```python
from build123d import *

# Parameters (mm, degrees)
BOX018_W     = 173
BOX018_H     = 97.5
BOX018_DEPTH = 30
BOX019_W     = 181
BOX019_H     = 121
BOX019_DEPTH = 5
BOX017_W     = 186
BOX017_H     = 127
BOX017_DEPTH = 2
FILLET008_R  = 2
FILLET009_R  = 1


with BuildPart() as cutout:
    # Box018 → Box018 (new body)
    with BuildSketch(Plane(origin=(6.5, 11, -25), x_dir=(1, 0, 0), z_dir=(0, 0, 1))):
        with Locations((86.5, 48.75)):
            Rectangle(BOX018_W, BOX018_H)
    extrude(amount=BOX018_DEPTH)


with BuildPart() as cube016:
    # Box019 → Box019 (new body)
    with BuildSketch(Plane(origin=(2.5, 3, -5), x_dir=(1, 0, 0), z_dir=(0, 0, 1))):
        with Locations((90.5, 60.5)):
            Rectangle(BOX019_W, BOX019_H)
    extrude(amount=BOX019_DEPTH)


with BuildPart() as fascia:
    # Box017 → Box017 (new body)
    with BuildSketch(Plane.XY):
        with Locations((93, 63.5)):
            Rectangle(BOX017_W, BOX017_H)
    extrude(amount=BOX017_DEPTH)

    # Fusion007: union Cube016
    add(cube016.part)

    # Cut007: cut Cutout
    add(cutout.part, mode=Mode.SUBTRACT)

    # Fillet008
    fillet008_edges = [fascia.edges().sort_by_distance(p)[0] for p in [
        (2.5, 124, -2.5),
        (2.5, 63.5, -5),
        (93, 3, -5),
        (183.5, 63.5, -5),
    ]]
    fillet(fillet008_edges, radius=FILLET008_R)

    # Fillet009
    fillet009_edges = [fascia.edges().sort_by_distance(p)[0] for p in [
        (2.973408, 123.292098, -4.292098),
        (93, 3, -3),
        (183.5, 124, -1.5),
        (0, 0, 1),
        (0, 127, 1),
        (186, 127, 1),
        (186, 0, 1),
        (186, 63.5, 2),
    ]]
    fillet(fillet009_edges, radius=FILLET009_R)


solid = fascia.part
```
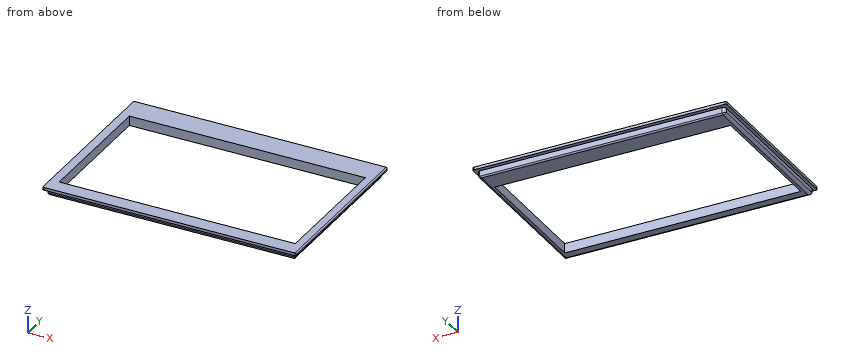
Source: CAD feature listing. Evaluate the final solid. Frame: model axes, mm. Coordinates: 2 decimals unless noted, no trailing zeros. Loops run counter-clockwise (first coordinate to the right, second up) from the corner with the lowest first, then second, coordinate; pieces in that order, holes last. Notation, with made-up numbers: (47.25, 56.25) -> (70.25, 56.25) arc R17 ccw to (70.25, 83.25) -> close; hole circle Ø2 at (70.5, 2.25). An arc over 180 degrees is marked (long way). One line per item, written item: value. Start each with the question number.
Q1. Contact query for flat-ended pins moving along their axis: P1, Ø1.2, axis at x = 86, z = -2.5, coming from the +Y side; P2, Ø1.5, axis at x = 42.5, z = -2, coming from the -Y side; P3, Ø2.5, axis at y = 81.5, z = -2, coming from the -X side. Output: stop coordinate, or through.
Q2. Line query: line 1 along X through (y, z) = (12.5, -3.25); line 2 along Y through (x, z) = (87.5, -0.25); line 3 along Y through (x, z) = (107, 0.75). Output: solid intervals per line, ascending.
Q3. Section query A-A, the plane x = 169. Return the cut outline in (y, z), and give its area (3 significant figures).
Q4. Section query B-B, the plane y = 95. Return the cut outline in (x, z).
Results:
1. P1: y = 124
1. P2: y = 3
1. P3: x = 2.5
2. line 1: 2.52 to 6.5, 179.5 to 183.48
2. line 2: 3 to 11, 108.5 to 124
2. line 3: 0 to 11, 108.5 to 127
3. outline: (0, 0) -> (3, 0) -> (3, -3) arc R2 ccw to (5, -5) -> (11, -5) -> (11, 2) -> (0, 2) -> close; (108.5, -5) -> (123, -5) arc R1 ccw to (124, -4) -> (124, 0) -> (127, 0) -> (127, 2) -> (108.5, 2) -> close
3. area: 175 mm^2
4. outline: (0, 0) -> (2.5, 0) -> (2.5, -3) arc R2 ccw to (4.5, -5) -> (6.5, -5) -> (6.5, 2) -> (0, 2) -> close; (179.5, -5) -> (181.5, -5) arc R2 ccw to (183.5, -3) -> (183.5, 0) -> (186, 0) -> (186, 1) arc R1 ccw to (185, 2) -> (179.5, 2) -> close
